For this review, take the finished solid that the model builds, in its own axes (mm). A direction names the side the tool comes from. Coordinates: 2 decimals unless noted, no trailing zeros. Loops run counter-clockwise (first coordinate to the right, second up) from the corner with the lowest first, then second, coordinate; pieces in that order, holes last. Notation, with made-up numbers: (14, 14.25) -> (32, 14.25) arc R14 cw to (32, 27.25) -> close; hole circle Ø5 at (24, 64.25). An arc over 180 degrees is marked (long way). Answer in a Markdown table with one row per item.
Autodesk Inventor part; units mm, degrees
ref_plane "YZ Plane" through (0, 0, 0) normal (1, 0, 0) x (0, 1, 0)
ref_plane "XZ Plane" through (0, 0, 0) normal (0, 1, 0) x (-1, 0, 0)
ref_plane "XY Plane" through (0, 0, 0) normal (0, 0, 1) x (1, 0, 0)
sketch "Boceto1" plane through (0, 0, 0) normal (0, 1, 0) x (-1, 0, 0)
  line L0 (0, 0) -> (0, -150)
  line L1 (0, -150) -> (-150, -150)
  line L2 (-150, -150) -> (-150, 0)
  line L3 (-150, 0) -> (0, 0)
extrude "Extrusión1" add sketch "Boceto1" along normal blind 4
sketch "Boceto2" plane through (0, 4, 0) normal (0, 1, 0) x (1, 0, 0)
  line L0 (0, 150) -> (4, 150)
  line L1 (150, 150) -> (0, 150)
  line L2 (0, 150) -> (0, 0)
  line L3 (0, 0) -> (150, 0)
  line L4 (150, 0) -> (150, 150)
  line L5 (0, 150) -> (150, 150)
  line L6 (4, 4) -> (146, 4)
  line L7 (146, 146) -> (146, 4)
  line L8 (146, 146) -> (4, 146)
  line L9 (4, 4) -> (4, 146)
extrude "Extrusión2" add sketch "Boceto2" along normal blind 46
sketch "Boceto3" plane through (0, 0, 0) normal (0, 0, 1) x (1, 0, 0)
  point P0 (0, 0)
sketch "Boceto4" plane through (0, 50, 0) normal (0, 1, 0) x (1, 0, 0)
  line L0 (4, 146) -> (146, 146)
  line L1 (0, 0) -> (0, 150)
  line L2 (146, 4) -> (4, 4)
  line L3 (2.3, 4) -> (2.3, 147.7)
  line L4 (2.3, 4) -> (2.3, 2.3)
  line L5 (2.3, 2.3) -> (147.7, 2.3)
  line L6 (147.7, 147.7) -> (2.3, 147.7)
  line L7 (147.7, 147.7) -> (147.7, 2.3)
  line L8 (4, 146) -> (146, 146)
  line L9 (146, 146) -> (146, 4)
  line L10 (146, 4) -> (146, 146)
  line L11 (4, 146) -> (4, 4)
  line L12 (4, 4) -> (146, 4)
extrude "Extrusión3" add sketch "Boceto4" along normal blind 7
sketch "Boceto5" plane through (0, 0, -150) normal (-1, 0, 0) x (0, 0, 1)
  point P0 (150, 0)
sketch "Boceto6" plane through (0, 0, -150) normal (-1, 0, 0) x (0, 0, 1)
  line L0 (0, 0) -> (0, 50)
  line L1 (0, 50) -> (4, 50)
  line L2 (0, 50) -> (150, 50)
  line L3 (146, 4) -> (4, 4)
  line L4 (4, 4) -> (4, 50)
  line L5 (4, 4) -> (146, 4)
  line L6 (146, 4) -> (146, 57)
  line L7 (146, 4) -> (146, 50)
  line L8 (146, 50) -> (4, 50)
  line L9 (147.7, 50) -> (2.3, 50)
  point P0 (150, 0)
extrude "Extrusión4" cut sketch "Boceto6" against normal blind 4
sketch "Boceto7" plane through (2.3, 50, -2.3) normal (-1, 0, 0) x (0, 0, 1)
  line L0 (-1.7, -46) -> (-1.7, 7)
  line L1 (-1.7, 0) -> (-1.7, 7)
  line L2 (-143.7, -46) -> (-143.7, 7)
  line L3 (-1.7, 7) -> (-143.7, 7)
  line L4 (-143.7, 7) -> (-143.7, 0)
  line L5 (2.3, 0) -> (-147.7, 0)
  line L6 (-143.7, 0) -> (-1.7, 0)
  point P0 (2.3, -50)
extrude "Extrusión5" cut sketch "Boceto7" against normal blind 4
sketch "Boceto8" plane through (0, 4, 0) normal (0, 1, 0) x (1, 0, 0)
  line L0 (0, 88.1) -> (106.1, 88.1)
  line L1 (106.1, 88.1) -> (106.1, 146)
  line L2 (0, 4) -> (0, 146)
  line L3 (0, 88.1) -> (0, 90.1)
  line L4 (2, 90.1) -> (104.1, 90.1)
  line L5 (106.1, 88.1) -> (104.1, 88.1)
  line L6 (104.1, 90.1) -> (104.1, 144)
  line L7 (106.1, 146) -> (106.1, 144)
  line L8 (104.1, 144) -> (2, 144)
  line L9 (0, 146) -> (106.1, 146)
  line L10 (2, 144) -> (2, 142)
  line L11 (2, 142) -> (0, 142)
  line L12 (2, 90.1) -> (2, 92.1)
  line L13 (2, 92.1) -> (0, 92.1)
  line L14 (0, 146) -> (0, 142)
  line L15 (0, 92.1) -> (0, 88.1)
  line L16 (2, 144) -> (2, 142)
  line L17 (2, 92.1) -> (2, 90.1)
  line L18 (0, 52) -> (48, 52)
  line L19 (48, 52) -> (48, 4)
  line L20 (0, 4) -> (146, 4)
  line L21 (2.3, 4) -> (0, 4)
  line L22 (0, 4) -> (48, 4)
  line L23 (2.3, 2.3) -> (147.7, 2.3)
  line L24 (0, 52) -> (0, 50)
  line L25 (2, 50) -> (46, 50)
  line L26 (46, 50) -> (46, 6)
  line L27 (46, 6) -> (2, 6)
  line L28 (0, 4) -> (48, 4)
  line L29 (0, 4) -> (48, 4)
  line L30 (2, 6) -> (2, 8)
  line L31 (2, 8) -> (0, 8)
  line L32 (2, 50) -> (2, 48)
  line L33 (2, 48) -> (0, 48)
  line L34 (2, 6) -> (2, 8)
  line L35 (2, 48) -> (2, 50)
  line L36 (0, 4) -> (0, 8)
  line L37 (0, 48) -> (0, 52)
  line L38 (0, 142) -> (0, 146)
  line L39 (0, 146) -> (106.1, 146)
  line L40 (2.3, 146) -> (146, 146)
  line L41 (106.1, 146) -> (106.1, 88.1)
  line L42 (106.1, 88.1) -> (0, 88.1)
  line L43 (0, 88.1) -> (0, 92.1)
  line L44 (0, 92.1) -> (2, 92.1)
  line L45 (2, 92.1) -> (2, 90.1)
  line L46 (2, 90.1) -> (104.1, 90.1)
  line L47 (104.1, 90.1) -> (104.1, 144)
  line L48 (104.1, 144) -> (2, 144)
  line L49 (2, 144) -> (2, 142)
  line L50 (2, 142) -> (0, 142)
  line L51 (0, 146) -> (2.3, 146)
  line L52 (0, 142) -> (0, 146)
  point P0 (0, 0)
extrude "Extrusión6" add sketch "Boceto8" along normal blind 2 contours L18 L19 L20 L2 L31 L30 L27 L26 L25 L32 L33
sketch "Boceto9" plane through (0, 4, 0) normal (0, 1, 0) x (1, 0, 0)
  line L0 (0, 88.1) -> (106.1, 88.1)
  line L1 (106.1, 88.1) -> (106.1, 146)
  line L2 (0, 88.1) -> (0, 90.1)
  line L3 (2, 90.1) -> (104.1, 90.1)
  line L4 (106.1, 88.1) -> (104.1, 88.1)
  line L5 (104.1, 90.1) -> (104.1, 144)
  line L6 (106.1, 146) -> (106.1, 144)
  line L7 (104.1, 144) -> (2, 144)
  line L8 (0, 146) -> (106.1, 146)
  line L9 (2, 144) -> (2, 142)
  line L10 (2, 142) -> (0, 142)
  line L11 (2, 90.1) -> (2, 92.1)
  line L12 (2, 92.1) -> (0, 92.1)
  line L13 (0, 146) -> (0, 142)
  line L14 (0, 92.1) -> (0, 88.1)
  line L15 (2, 144) -> (2, 142)
  line L16 (2, 92.1) -> (2, 90.1)
  line L17 (0, 142) -> (0, 146)
  line L18 (0, 146) -> (106.1, 146)
  line L19 (106.1, 146) -> (106.1, 88.1)
  line L20 (106.1, 88.1) -> (0, 88.1)
  line L21 (0, 88.1) -> (0, 92.1)
  line L22 (0, 92.1) -> (2, 92.1)
  line L23 (2, 92.1) -> (2, 90.1)
  line L24 (2, 90.1) -> (104.1, 90.1)
  line L25 (104.1, 90.1) -> (104.1, 144)
  line L26 (104.1, 144) -> (2, 144)
  line L27 (2, 144) -> (2, 142)
  line L28 (2, 142) -> (0, 142)
  line L29 (0, 146) -> (2.3, 146)
  line L30 (0, 142) -> (0, 146)
  point P0 (0, 0)
  point P1 (0, 52)
extrude "Extrusión7" add sketch "Boceto9" along normal blind 2
properties part number "base inf"
Item 1: For faces 1 (the flat face through (74, 53, -2.3)), 2 (the flat face through (53, 6, -89)), 3 (the flat face through (147.7, 53, -76)), 4 (the flat face through (76, 53, -147.7)), list the 3-axis set-ups (+Z, -Z, +X, -X, +Y, -Y) from which the entire face can be reached by the end or side of a thin tool; tool diameter is ignored.
Worked answers:
| item | result |
|---|---|
| face 1 | +Z, +X, -X, +Y |
| face 2 | -X, +Y |
| face 3 | +Z, -Z, +X, +Y |
| face 4 | -Z, +X, -X, +Y |
Item 2: For L1, parallel to Z at x = 104, y = 4.5; L2, parallel to Z at x = 35, y = 49; L3, parallel to Y at x = 81, z = -8, list the stretches that pass through material, from the lowest coordinate up.
Worked answers:
| item | result |
|---|---|
| L1 | -150 to -144, -90.1 to -88.1, -4 to 0 |
| L2 | -150 to -146, -4 to 0 |
| L3 | 0 to 4 |
Item 3: Take a section at A-A, the plane z = -44. State the section outline as (x, y) points, and give its area (3 significant figures).
Worked answers:
| item | result |
|---|---|
| outline | (0, 0) -> (150, 0) -> (150, 50) -> (147.7, 50) -> (147.7, 57) -> (146, 57) -> (146, 4) -> (48, 4) -> (48, 6) -> (46, 6) -> (46, 4) -> (0, 4) -> close |
| area | 800 mm² |
Item 4: The part is to be moulded in two halves that separate along X. For faces 5 (the flat face through (88, 4, -58)), 6 (the flat face through (0, 3, -69)), 7 (the flat face through (150, 25, -76)), 8 (the flat face through (74, 25, -150)), say which applies: +X half, -X half, draft (parallel to the pull), parting line (faces both ways), or undercut.
Worked answers:
| item | result |
|---|---|
| face 5 | undercut |
| face 6 | -X half |
| face 7 | +X half |
| face 8 | draft |
Item 5: Insertion check: pin 1 (5 mm diameter, centred on x = 85.5, z = -31, fed in from +Y); pin 2 (5 mm diameter, centred on y = 15, z = -63, fed in from -X); pin 3 (0.5 mm diameter, centred on y = 54, z = -147, fed in from -X). Each pin has a flat end and moves straight along its axis. Give the tip position at first contact, or say it passes through.
Worked answers:
| item | result |
|---|---|
| pin 1 | y = 4 |
| pin 2 | x = 146 |
| pin 3 | x = 2.3 |
Item 6: Take a section at B-B, the plane y = 29. State the section outline as (x, z) points, and give its area (3 significant figures).
Worked answers:
| item | result |
|---|---|
| outline | (0, -150) -> (150, -150) -> (150, 0) -> (0, 0) -> (0, -4) -> (146, -4) -> (146, -146) -> (0, -146) -> close |
| area | 1,770 mm² |
Item 7: Take a section at D-D, the plane z = -81. State the section outline as (x, y) points, and give its area (3 significant figures).
Worked answers:
| item | result |
|---|---|
| outline | (0, 0) -> (150, 0) -> (150, 50) -> (147.7, 50) -> (147.7, 57) -> (146, 57) -> (146, 4) -> (0, 4) -> close |
| area | 796 mm² |
Item 8: Take a section at C-C, the plane x = 74. State the section outline as (y, z) points, and give its area (4 significant figures).
Worked answers:
| item | result |
|---|---|
| outline | (0, -150) -> (50, -150) -> (50, -147.7) -> (57, -147.7) -> (57, -146) -> (6, -146) -> (6, -144) -> (4, -144) -> (4, -90.1) -> (6, -90.1) -> (6, -88.1) -> (4, -88.1) -> (4, -4) -> (57, -4) -> (57, -2.3) -> (50, -2.3) -> (50, 0) -> (0, 0) -> close |
| area | 1,000 mm² |
